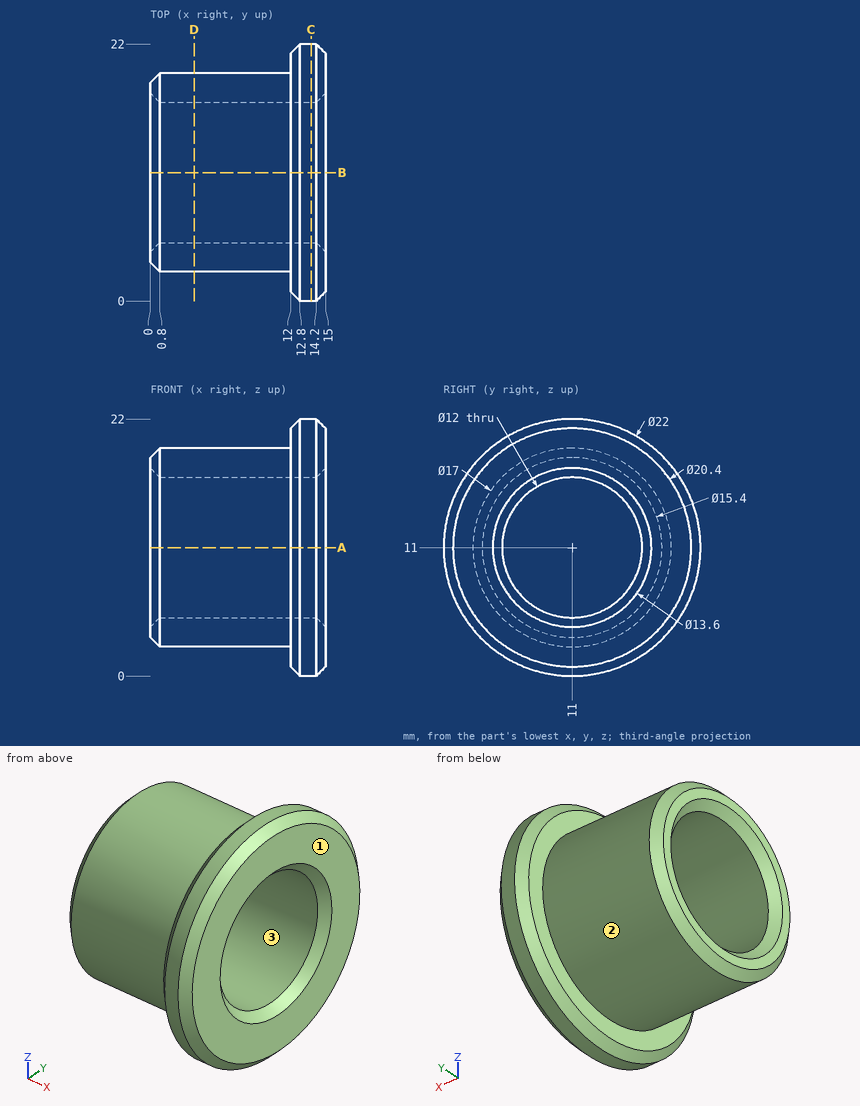
Can you work these out from the drawing? Everything is in mm from the part's minimum corner. Round coordinates to 2 decimals unless told otherwise and drop trailing zeros. Write each loop counter-clockwise with the first axis right and the second up, starting at its lowest first coordinate (ties: lowest second). Pieces come first, ordered by that corner, then holes. Notation, with made-up numbers: M 54,37.25 L 113,37.25 A30 ccw 113,64.25 Z; hole C 89,54.25 d7. An arc over 180 degrees is marked long. Use a Markdown table: item, result.
Item 1: I want a section at C-C (x = 13.75). List the corners of the cut face in (y, z) for me, and give its area (3 significant figures).
Found:
| item | result |
|---|---|
| outline | C 11,11 d22; hole C 11,11 d12 |
| area | 267 mm2 |
Item 2: I want a section at A-A (z = 11). List the corners of the cut face in (x, y) for me, and give its area (3 significant figures).
Found:
| item | result |
|---|---|
| outline | M 0,3.3 L 0.8,2.5 L 12,2.5 L 12,0.8 L 12.8,0 L 14.2,0 L 15,0.8 L 15,4.2 L 14.2,5 L 0.8,5 L 0,4.2 Z; M 0,17.8 L 0.8,17 L 14.2,17 L 15,17.8 L 15,21.2 L 14.2,22 L 12.8,22 L 12,21.2 L 12,19.5 L 0.8,19.5 L 0,18.7 Z |
| area | 86.8 mm2 |
Item 3: For pin 1 Ø2 at (x, y) = (3, 10) entering from +Z; pin 2 Ø1 at (x, y) = (5.5, 13) entering from -Z; pin 3 Ø5 at (x, z) = (8.5, 15.5) entering from +Y, each with a flat end and sliding along its axis, tell me the tip position at first contact or that it passes through.
Found:
| item | result |
|---|---|
| pin 1 | stops at z = 19.5 |
| pin 2 | stops at z = 2.63 |
| pin 3 | stops at y = 19.26 |
Item 4: If I drill on line 1 along Y through (x, z) = (10.75, 11); line 2 along Y through (x, z) = (8, 16), over which ranges is the centre line in solid material (lowest first)? Write a range as [from, to].
Found:
| item | result |
|---|---|
| line 1 | y = [2.5, 5], [17, 19.5] |
| line 2 | y = [4.13, 7.68], [14.32, 17.87] |
Item 5: We'd pull the mould along Y, two halves only. Please class the marked faces 1, 2 and 3: released by +Y, released by -Y, zero draft, split by the parting line, or undercut.
Found:
| item | result |
|---|---|
| face 1 | zero draft |
| face 2 | split by the parting line |
| face 3 | undercut |
Item 6: I want a section at D-D (x = 3.75). List the corners of the cut face in (y, z) for me, and give its area (3 significant figures).
Found:
| item | result |
|---|---|
| outline | C 11,11 d17; hole C 11,11 d12 |
| area | 114 mm2 |
